```python
from build123d import *

# Parameters (mm, degrees)
F0_W     = 12.7
F0_H     = 76.2
F1_DEPTH = 11.43


# Not quite as in the source:
# - a feature names something its author has since deleted; it is built from what else it names


with BuildPart() as f1:
    # F0 (on Front) → F1 (new body)
    with BuildSketch(Plane.XZ):
        with BuildLine():
            Line((86.44143009, 487.5982903777), (-82.6555196025, 487.5982903777))
            Line((-82.6555196025, 487.5982903777), (-18.7736136836, 426.7721436688))
            ThreePointArc((-18.7736136836, 426.7721436688), (-15.8484759418, 383.977401572), (-58.2239000145, 377.323844885))
            Line((-58.2239000145, 377.323844885), (-104.05856991, 407.7417460511))
            Line((-104.05856991, 407.7417460511), (-104.05856991, -133.2205747848))
            Line((-104.05856991, -133.2205747848), (-23.008097061, -186.9833762889))
            ThreePointArc((-23.008097061, -186.9833762889), (-14.1002365767, -230.9921824712), (-58.109042759, -239.9000429556))
            Line((-58.109042759, -239.9000429556), (-104.05856991, -209.4205747848))
            Line((-104.05856991, -209.4205747848), (-104.05856991, -346.656112826))
            Line((-104.05856991, -346.656112826), (-23.121974943, -400.3433762889))
            ThreePointArc((-23.121974943, -400.3433762889), (-14.2141144586, -444.3521824712), (-58.2229206409, -453.2600429556))
            Line((-58.2229206409, -453.2600429556), (-104.05856991, -422.856112826))
            Line((-104.05856991, -422.856112826), (-104.05856991, -477.484384418))
            Line((-104.05856991, -477.484384418), (-22.7666009966, -531.4073762889))
            ThreePointArc((-22.7666009966, -531.4073762889), (-13.8587405122, -575.4161824712), (-57.8675466945, -584.3240429556))
            Line((-57.8675466945, -584.3240429556), (-104.05856991, -553.684384418))
            Line((-104.05856991, -553.684384418), (-104.05856991, -575.4260893394))
            Line((-104.05856991, -575.4260893394), (-23.5744710882, -625.3769093504))
            ThreePointArc((-23.5744710882, -625.3769093504), (-13.5964073743, -669.50213472), (-57.8674036509, -678.8121378395))
            Line((-57.8674036509, -678.8121378395), (-104.05856991, -648.172744022))
            Line((-104.05856991, -648.172744022), (-104.05856991, -711.2817096223))
            Line((-104.05856991, -711.2817096223), (47.07143009, -711.2817096223))
            Line((47.07143009, -711.2817096223), (86.44143009, -711.2817096223))
            Line((86.44143009, -711.2817096223), (86.44143009, 487.5982903777))
        make_face()
        with Locations((47.07143009, -642.7017096223)):
            Rectangle(F0_W, F0_H, mode=Mode.SUBTRACT)
        with Locations((47.07143009, -210.3231889248)):
            Rectangle(F0_W, F0_H, mode=Mode.SUBTRACT)
    extrude(amount=F1_DEPTH)


solid = f1.part
```
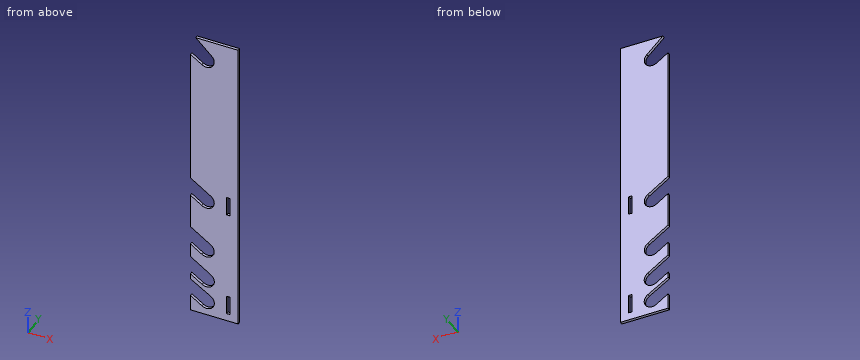
Here's how the part is built. I have some questions about the finished solid (model axes, mm). Round coordinates to 2 decimals unless told otherwise and drop trailing zeros. Write each loop counter-clockwise with the first axis right and the second up, starting at its lowest first coordinate (ties: lowest second). Pieces come first, ordered by that corner, then holes.
Q1. If we section it at A-A on y = -6: Give the number of separate pieces and of enclosed holes in the cut face, plus the area to 3 significant figures.
Q2. Will this pin go through, and if not, where does the flat tip stop? P1, Ø3.5, axis at y = -4, z = -639.5, coming from the -X side (3 decimals).
Q3. If we section it at C-C on z = -435: Write out the boundary of the cut face in (x, y).
Q4. If we section it at B-B on x = -41: Write out the boundary of the cut face in (y, z), plus the area to 3 significant figures.
Q5. Please list where these lines run through material, in increasing order: probe 1 along Z at (x, y) = (-74, -3.5); probe 2 along Z at (x, y) = (-95.5, -7.5); probe 3 along Z at (x, y) = (-72, -10.5).
Answer below:
1. separate pieces: 1
1. enclosed holes: 2
1. area: 194,000 mm2
2. P1: stops at x = -12.125
3. outline: (-104.06, -11.43) - (-85.75, -11.43) - (-85.75, 0) - (-104.06, 0) - close; (-10, -11.43) - (86.44, -11.43) - (86.44, 0) - (-10, 0) - close
4. outline: (-11.43, -711.28) - (0, -711.28) - (0, -684.1) - (-11.43, -684.1) - close; (-11.43, -614.56) - (0, -614.56) - (0, -589.61) - (-11.43, -589.61) - close; (-11.43, -519.31) - (0, -519.31) - (0, -458.55) - (-11.43, -458.55) - close; (-11.43, -388.48) - (0, -388.48) - (0, -245.19) - (-11.43, -245.19) - close; (-11.43, -175.05) - (0, -175.05) - (0, 372.03) - (-11.43, 372.03) - close; (-11.43, 447.94) - (0, 447.94) - (0, 487.6) - (-11.43, 487.6) - close
4. area: 9,630 mm2
5. probe 1: z = -711.28 to -668.11, -594.08 to -573.62, -497.42 to -442.79, -366.59 to -229.36, -153.16 to 387.79, 479.36 to 487.6
5. probe 2: z = -711.28 to -653.85, -580.74 to -559.36, -483.16 to -428.53, -352.33 to -215.1, -138.9 to 402.06
5. probe 3: z = -711.28 to -669.44, -595.32 to -574.95, -498.75 to -444.12, -367.92 to -230.69, -154.49 to 386.47, 477.45 to 487.6
